from build123d import *

# Parameters (mm, degrees)
F0_W     = 38.1
F0_H     = 76.2
F1_DEPTH = 444.5
F2_W     = 21.9964
F2_H     = 38.1
F3_DEPTH = 6.35


with BuildPart() as f1:
    # F0 (on Right) → F1 (new body, symmetric)
    with BuildSketch(Plane.YZ):
        Rectangle(F0_W, F0_H)
    extrude(amount=F1_DEPTH, both=True)

    # F2 (on face) → F3 (cut)
    with BuildSketch(Plane(origin=(0, 0, -38.1), x_dir=(1, 0, 0), z_dir=(0, 0, -1))):
        with Locations((393.7, 0)):
            Rectangle(F2_W, F2_H)
        with Locations((-393.7, 0)):
            Rectangle(F2_W, F2_H)
    extrude(amount=-F3_DEPTH, mode=Mode.SUBTRACT)


solid = f1.part
Design review of the part built by this model. Coordinates are the model's own, in mm. A direction names the side the tool comes from. Give positions to 0.01 mm unless a question says otherwise; leave off trailing zeros.
1. For pin 1 Ø11 at (x, y) = (-394, 3.5) entering from -Z, flat-tipped, find the tip position at first contact; note if it passes through.
Solution:
pin 1: stops at z = -31.75
2. To check wall thickness, follow L1, parallel to Z at x = -396.5, y = 11.5. State the ranges of the line that lie inside material, in increasing order.
Solution:
L1: z = -31.75 to 38.1
3. Mouldability with a two-part tool opening along X and no side actions: class faces 3 (the flat face through (6, 19.05, -1)), 4 (the flat face through (-444.5, 0, 1)), 5 (the flat face through (444.5, 0, 1)), 6 (the flat face through (-394, 0, -31.75)) as +X half, -X half, draft (parallel to the pull), parting line (faces both ways), or undercut.
Solution:
face 3: draft
face 4: -X half
face 5: +X half
face 6: undercut
4. Tool access review of faces 1 (the flat face through (394, 0, -31.75)), 2 (the flat face through (-424, 0, -38.1)): name each direction out of +Z, -Z, +X, -X, +Y, -Y from which nothing blocks a thin tool from reaching the whole face with its end or side.
Solution:
face 1: -Z, +Y, -Y
face 2: -Z, +X, -X, +Y, -Y
